```python
from build123d import *

# Parameters (mm, degrees)
F0_W     = 152.4
F0_H     = 76.2
F1_DEPTH = 25.4
F2_R     = 8.89
F2_R_2   = 9.33931
F2_R_3   = 9.03456
F2_R_4   = 9.786488
F3_DEPTH = 50.8
F4_W     = 12.7
F4_H     = 50.8


with BuildPart() as f1:
    # F0 (on Top) → F1 (new body)
    with BuildSketch(Plane.XY):
        Rectangle(F0_W, F0_H)
    extrude(amount=-F1_DEPTH)

    # F2 (on Top) → F3 (cut)
    with BuildSketch(Plane.XY):
        with Locations((-64.024046, 23.457246)):
            Circle(F2_R)
        with Locations((63.710019, 26.510652)):
            Circle(F2_R_2)
        with Locations((-63.006245, -23.870517)):
            Circle(F2_R_3)
        with Locations((64.218916, -24.379414)):
            Circle(F2_R_4)
    extrude(amount=-F3_DEPTH, mode=Mode.SUBTRACT)

    # F4 (on Front) → F5 (revolve)
    with BuildSketch(Plane.XZ):
        with Locations((6.35, 25.4)):
            Rectangle(F4_W, F4_H)
    revolve(axis=Axis((0, 0, 25.4), (0, 0, 1)))


solid = f1.part
```
Geometry check sheet. Reference: the model listing, model coordinates, mm. A direction names the side the tool comes from. Coordinates: 2 decimals unless noted, no trailing zeros. Order: outer loops, then holes, each group sorted by start corner. A loop starts at its lowest first (then second) coordinate and runs counter-clockwise, first axis right, second up.
Q1. Depth check by flat-ended pin: pin 1 Ø11 at (x, y) = (-63.01, -23.87) entering from +Z; pin 2 Ø8 at (x, y) = (-25.5, 20) entering from +Z. Enter the tip coordinate at first touch or a pass-through.
Reply:
pin 1: passes through
pin 2: stops at z = 0
Q2. Draft check along X on faces 1 (the face through (-1, 1, -25.4)), 2 (the face through (-58.837, -31.886, -12.522)), 3 (the face through (-76.2, -1, -13)). Enter one of: released by +X, released by -X, zero draft, split by the parting line, or undercut.
Reply:
face 1: zero draft
face 2: undercut
face 3: released by -X
Q3. Tool access check on faces 4 (the face through (0, 0, 50.8)), 5 (the face through (-2.75, -12.4, 25.76)). Record the directions out of +Z, -Z, +X, -X, +Y, -Y that give a thin tool (end or side, any length) a straight path to the whole face; none if there is none.
Reply:
face 4: +Z, +X, -X, +Y, -Y
face 5: +Z
Q4. Sectioned sample at A-A on x = 0. Record the cut outline in (y, z), and give its area (3 significant figures).
Reply:
outline: (-38.1, -25.4) - (38.1, -25.4) - (38.1, 0) - (12.7, 0) - (12.7, 50.8) - (-12.7, 50.8) - (-12.7, 0) - (-38.1, 0) - close
area: 3,230 mm2
Q5. Thickness scan on probe 1 along X at (y, z) = (-23.5, -6.5); probe 2 along X at (y, z) = (23.5, -11.5); probe 3 along Y at (x, z) = (70, -11.5). Record the ranges inside material, lowest first.
Reply:
probe 1: x = -76.2 to -72.03, -53.98 to 54.47, 73.97 to 76.2
probe 2: x = -76.2 to -72.91, -55.13 to 54.87, 72.55 to 76.2
probe 3: y = -38.1 to -32.28, -16.48 to 19.61, 33.41 to 38.1
Q6. Sectioned sample at B-B on y = -19. Record the cut outline in (x, z).
Reply:
outline: (-76.2, -25.4) - (-70.62, -25.4) - (-70.62, 0) - (-76.2, 0) - close; (-55.4, -25.4) - (56.04, -25.4) - (56.04, 0) - (-55.4, 0) - close; (72.39, -25.4) - (76.2, -25.4) - (76.2, 0) - (72.39, 0) - close
Q7. Sectioned sample at C-C on y = 0. Record the cut outline in (x, z), and give its area (3 significant figures).
Reply:
outline: (-76.2, -25.4) - (76.2, -25.4) - (76.2, 0) - (12.7, 0) - (12.7, 50.8) - (-12.7, 50.8) - (-12.7, 0) - (-76.2, 0) - close
area: 5,160 mm2
Q8. Sectioned sample at D-D on z = 25.5. Record the cut outline in (x, y).
Reply:
outline: circle Ø25.4 at (0, 0)
